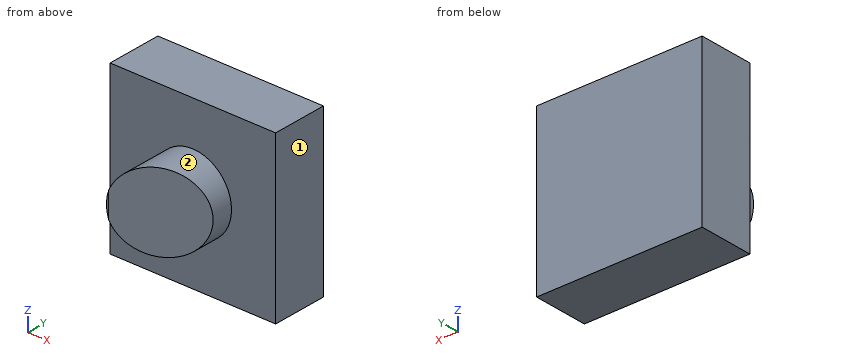
```python
from build123d import *

# Parameters (mm, degrees)
F0_W     = 38.1
F0_H     = 38.1
F1_DEPTH = 12.7
F2_R     = 8.89
F3_DEPTH = 12.7
F5_DEPTH = 254


with BuildPart() as f1:
    # F0 (on Front) → F1 (new body)
    with BuildSketch(Plane.XZ):
        with Locations((19.05, 19.05)):
            Rectangle(F0_W, F0_H)
    extrude(amount=F1_DEPTH)

    # F2 (on face) → F3 (join)
    with BuildSketch(Plane.XZ.offset(12.7)):
        with Locations((19.05, 19.05)):
            Circle(F2_R)
    extrude(amount=F3_DEPTH)

    # F4 (on Top) → F5 (cut)
    with BuildSketch(Plane.XY):
        Polygon((29.379437, -16.942142), (9.009695, -26.147699), (29.379437, -26.147699), align=None)
    extrude(amount=F5_DEPTH, mode=Mode.SUBTRACT)


solid = f1.part
```
CAD build for the part. Positions are in the model's coordinates, mm. Face numbers are marked on the shaded views. A direction names the side the tool comes from. Round coordinates to 2 decimals unless told otherwise and drop trailing zeros. Order: outer loops, then holes, each group sorted by start corner. A loop starts at its lowest first (then second) coordinate and runs counter-clockwise, first axis right, second up. Notation, with made-up numbers: (-27.75, -29) -> (-22.75, -29) arc R12 cw to (-22.75, -15) -> close; hole circle Ø10 at (44.25, 52.5). An arc over 180 degrees is marked (long way). Write item = value, one per line.
(1) 3-axis set-ups, long thin cutter, end or side, ignore diameter. For the marked faces 1 and 2: which of +Z, -Z, +X, -X, +Y, -Y reach the whole face in a straight line?
Answers follow:
face_1 = +Z, -Z, +X, +Y, -Y
face_2 = -Y
(2) Drill centre lines: L1, parallel to Y at x = 30, z = 20.5; L2, parallel to Y at x = 16.5, z = 25; L3, parallel to X at y = -19, z = 19.5. Where is each one in solid material? Low to high.
Answers follow:
L1 = -12.7 to 0
L2 = -22.76 to 0
L3 = 10.17 to 24.83
(3) Cut at D-D (z = 14.5). Write the cut outline in (x, y).
Answers follow:
outline = (0, -12.7) -> (11.41, -12.7) -> (11.41, -25.06) -> (26.69, -18.16) -> (26.69, -12.7) -> (38.1, -12.7) -> (38.1, 0) -> (0, 0) -> close
(4) Flat gauge pins, fed straight in: P1, Ø10, axis at x = 11.5, y = -20.5, coming from the -Z side; P2, Ø4, axis at x = 16.5, z = 27.5, coming from the -Y side; P3, Ø6, axis at x = 12, z = 20, coming from the +Y side; P4, Ø3, axis at x = 11.5, y = -21.5, coming from the +Z side. Where does each tip first touch, or does it go through?
Answers follow:
P1 = 10.53
P2 = -23.6
P3 = 0
P4 = 25.56
(5) Cut at A-A (z = 19.05). Write the cut outline in (x, y), plus the area to 3 significant figures.
Answers follow:
outline = (0, -12.7) -> (10.16, -12.7) -> (10.16, -25.4) -> (10.66, -25.4) -> (27.94, -17.59) -> (27.94, -12.7) -> (38.1, -12.7) -> (38.1, 0) -> (0, 0) -> close
area = 642 mm²
(6) Cut at B-B (x = 25). Write the cut outline in (y, z).
Answers follow:
outline = (-18.92, 12.44) -> (-12.7, 12.44) -> (-12.7, 0) -> (0, 0) -> (0, 38.1) -> (-12.7, 38.1) -> (-12.7, 25.66) -> (-18.92, 25.66) -> close
(7) Cut at C-C (y = -16.75). Write the cut outline in (x, z), plus the area to 3 significant figures.
Answers follow:
outline = circle Ø17.78 at (19.05, 19.05)
area = 248 mm²
